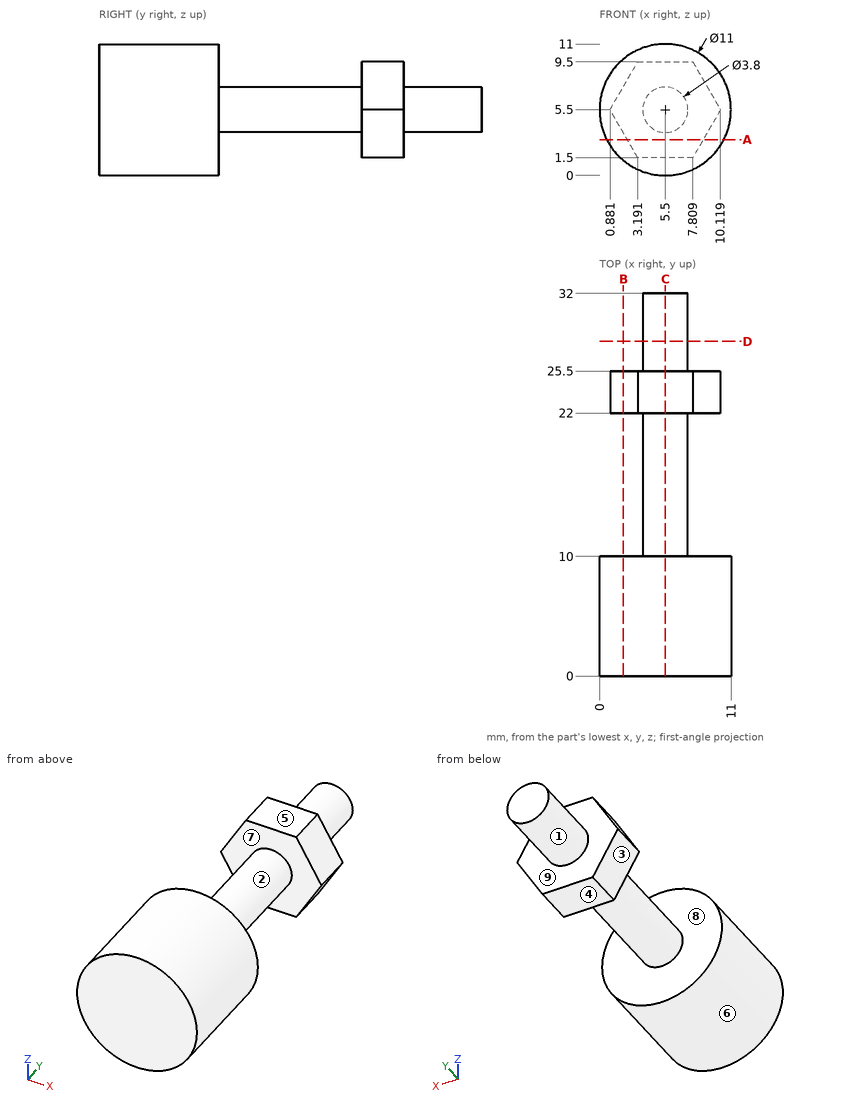
Could you check a few things on this drawing? It's one solid part, dimensions in mm from its lowest x, y, z. A direction names the side the tool comes from. Round coordinates to 2 decimals unless told otherwise and drop trailing zeros. Loops run counter-clockwise (first coordinate to the right, second up) from the corner with the lowest first, then second, coordinate; pieces in that order, holes last.
Q1. I want a section at C-C (x = 5.5). Write out the boundary of the cut face in (y, z).
Q2. For P1, Ø3, axis at x = 5.5, y = 23, coming from the +Z side; P2, Ø2, axis at y = 4.5, z = 9, coming from the +X side; P3, Ø1, axis at y = 5, z = 3, coming from the +X side, each with a flat end and sliding along its axis, tell me the tip position at first contact or that it passes through.
Q3. I want a section at D-D (y = 28). Write out the boundary of the cut face in (x, z).
Q4. Thinking about a two-plate mould opening in Y: for the marked faces 6, 7, 8 and 9, which applies, pulls with the +Y half, pulls with the -Y half, needs draft (parallel to the pull), parting line crosses it, or undercut?
Q5. Please list where these lines run through material, in increasing order: L1, parallel to Y at x = 2.75, z = 6.25; L2, parallel to Y at x = 10, z = 6.5; L3, parallel to Z at x = 5.5, y = 21.
Q6. I want a section at B-B (x = 2). Write out the boundary of the cut face in (y, z).
Q7. On a 3-axis mill with a long thin cutter (end or side, diameter ignored), from which of +Z, -Z, +X, -X, +Y, -Y can I reach the whole of each face in a straight line? I mean the marked faces 1, 2, 3, 4 and 5. Say none if no direction works.
Q8. I want a section at A-A (z = 3). Write out the boundary of the cut face in (x, y) (1 decimal), and give its area (3 significant figures).
Answer below:
1. outline: (0, 0) - (10, 0) - (10, 3.6) - (22, 3.6) - (22, 1.5) - (25.5, 1.5) - (25.5, 3.6) - (32, 3.6) - (32, 7.4) - (25.5, 7.4) - (25.5, 9.5) - (22, 9.5) - (22, 7.4) - (10, 7.4) - (10, 11) - (0, 11) - close
2. P1: stops at z = 9.5
2. P2: stops at x = 10.4
2. P3: stops at x = 10.62
3. outline: circle Ø3.8 at (5.5, 5.5)
4. face 6: needs draft
4. face 7: undercut
4. face 8: undercut
4. face 9: pulls with the +Y half
5. L1: y = 0 to 10, 22 to 25.5
5. L2: y = 0 to 10
5. L3: z = 3.6 to 7.4
6. outline: (0, 1.26) - (10, 1.26) - (10, 9.74) - (0, 9.74) - close; (22, 3.56) - (25.5, 3.56) - (25.5, 7.44) - (22, 7.44) - close
7. face 1: +Y
7. face 2: none
7. face 3: -Z, -X, +Y
7. face 4: -Z, +X, -X, +Y
7. face 5: +Z, +X, -X, +Y
8. outline: (0.6, 0) - (10.4, 0) - (10.4, 10) - (0.6, 10) - close; (2.3, 22) - (8.7, 22) - (8.7, 25.5) - (2.3, 25.5) - close
8. area: 120 mm2
